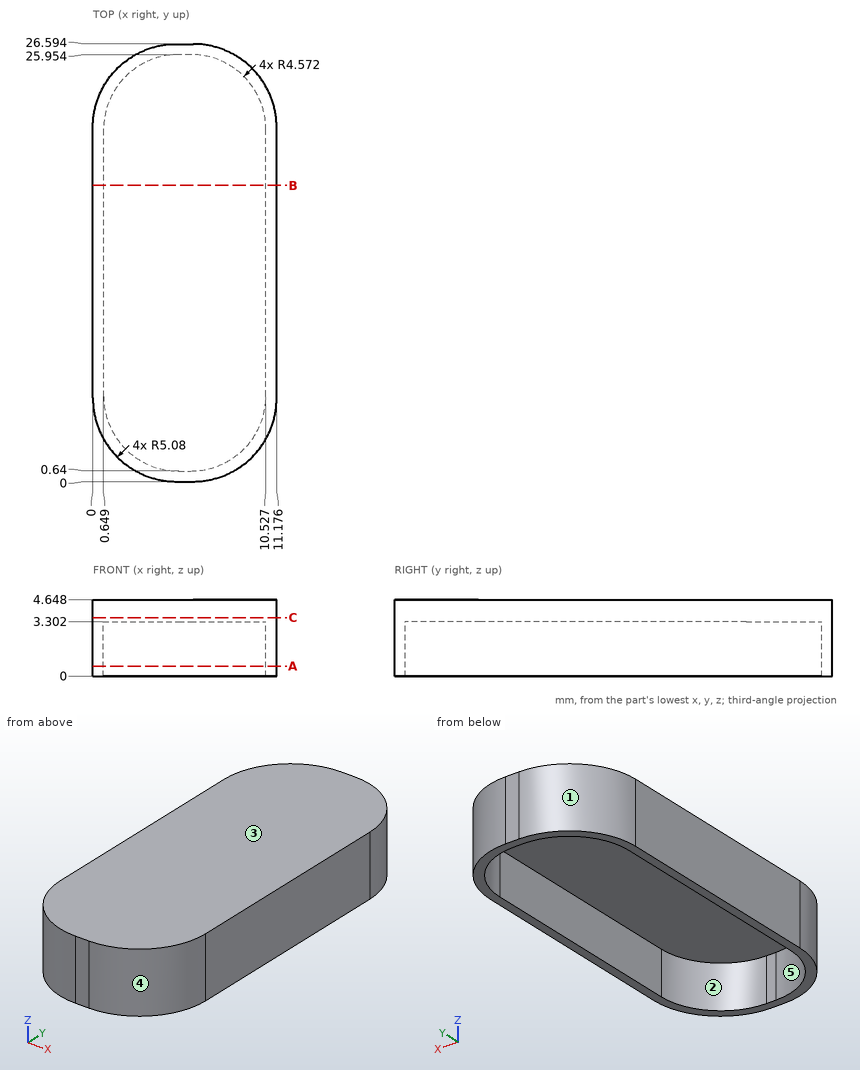
The figure shows three views and two pictorial views of one solid part (mm, origin at its lowest corner). Answer the questions. A direction names the side the tool comes from. Round coordinates to 2 decimals unless told otherwise and drop trailing zeros. Order: outer loops, then holes, each group sorted by start corner. A loop starts at its lowest first (then second) coordinate and runs counter-clockwise, first axis right, second up.
Q1. The mould has two halves that part along X. Classify the marked faces 3, 4 and 5: pulls with the +X half, pulls with the -X half, needs draft (parallel to the pull), parting line crosses it, or undercut.
Solution:
face 3: needs draft
face 4: pulls with the +X half
face 5: undercut
Q2. Given pin 1 Ø4 at (x, y) = (7, 10.5) entering from -Z; pin 2 Ø1.5 at (x, z) = (2.5, 1.5) entering from -Y, each flat-ended and moving along its own axis, determine where each tip first touches the part or whether it passes through.
Solution:
pin 1: stops at z = 3.3
pin 2: stops at y = 0.34
Q3. A tool of negligible diameter and unlimited length cuts with its end or side. For the marked faces 1 and 2, from which of +Z, -Z, +X, -X, +Y, -Y can it reach the whole face along a straight path? Write none if from no direction.
Solution:
face 1: +Z, -Z, -X, +Y
face 2: -Z
Q4. A cutting plane is placed at A-A, the plane z = 0.6. Determine the outline of the cut face in (x, y) (1 decimal).
Solution:
outline: (0, 5.1) arc R5.1 ccw to (5.1, 0) - (6.1, 0) arc R5.1 ccw to (11.2, 5.1) - (11.2, 21.5) arc R5.1 ccw to (6.1, 26.6) - (5.1, 26.6) arc R5.1 ccw to (0, 21.5) - close; hole (0.6, 5.2) arc R4.6 ccw to (5.2, 0.6) - (6, 0.6) arc R4.6 ccw to (10.5, 5.2) - (10.5, 21.4) arc R4.6 ccw to (6, 26) - (5.2, 26) arc R4.6 ccw to (0.6, 21.4) - close
Q5. Find the intervals of material crossed by line 1 along X through (y, z) = (14.5, 2.3); line 2 along Y through (x, z) = (6, 1.05); line 3 along Z through (x, y) = (8.25, 17), in increasing order.
Solution:
line 1: x = 0 to 0.65, 10.53 to 11.18
line 2: y = 0 to 0.64, 25.95 to 26.59
line 3: z = 3.3 to 4.65
Q6. A cutting plane is placed at C-C, the plane z = 3.55. Determine the outline of the cut face in (x, y), then the cut area to 3 significant figures.
Solution:
outline: (0, 5.08) arc R5.08 ccw to (5.08, 0) - (6.1, 0) arc R5.08 ccw to (11.18, 5.08) - (11.18, 21.51) arc R5.08 ccw to (6.1, 26.59) - (5.08, 26.59) arc R5.08 ccw to (0, 21.51) - close
area: 275 mm2
Q7. A cutting plane is placed at B-B, the plane y = 18. Determine the outline of the cut face in (x, z).
Solution:
outline: (0, 0) - (0.65, 0) - (0.65, 3.3) - (10.53, 3.3) - (10.53, 0) - (11.18, 0) - (11.18, 4.65) - (0, 4.65) - close
